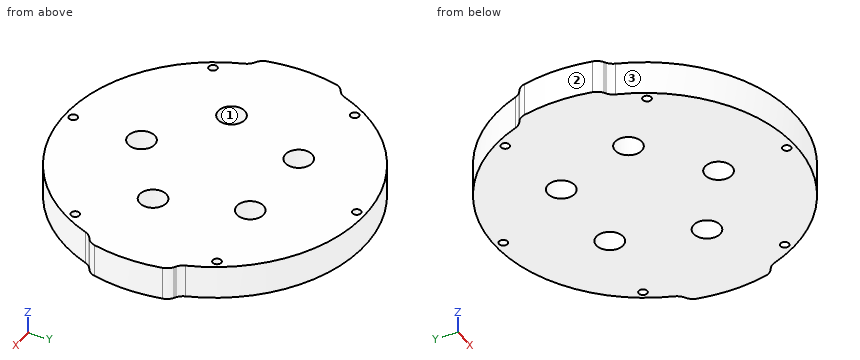
from build123d import *

# Parameters (mm, degrees)
SKETCH1_R           = 1.6
BOSS_EXTRUDE1_DEPTH = 12.7
SKETCH6_R           = 5.1
CUT_EXTRUDE2_DEPTH  = 13.7
FILLET1_R           = 5


with BuildPart() as part:
    # Sketch1 → Boss-Extrude1 (new body)
    with BuildSketch(Plane.XY):
        with BuildLine():
            Line((54.404710274, 17.5), (58.249656651, 15))
            ThreePointArc((58.249656651, 15), (60.15, 0), (58.249656651, -15))
            Line((58.249656651, -15), (54.404710274, -17.5))
            ThreePointArc((54.404710274, -17.5), (0, -57.15), (-54.404710274, -17.5))
            Line((-54.404710274, -17.5), (-58.249656651, -15))
            ThreePointArc((-58.249656651, -15), (-60.15, 0), (-58.249656651, 15))
            Line((-58.249656651, 15), (-54.404710274, 17.5))
            ThreePointArc((-54.404710274, 17.5), (0, 57.15), (54.404710274, 17.5))
        make_face()
        with Locations((0, 53.975)):
            Circle(SKETCH1_R, mode=Mode.SUBTRACT)
        with Locations((46.743721169, 26.9875)):
            Circle(SKETCH1_R, mode=Mode.SUBTRACT)
        with Locations((46.743721169, -26.9875)):
            Circle(SKETCH1_R, mode=Mode.SUBTRACT)
        with Locations((0, -53.975)):
            Circle(SKETCH1_R, mode=Mode.SUBTRACT)
        with Locations((-46.743721169, -26.9875)):
            Circle(SKETCH1_R, mode=Mode.SUBTRACT)
        with Locations((-46.743721169, 26.9875)):
            Circle(SKETCH1_R, mode=Mode.SUBTRACT)
    extrude(amount=BOSS_EXTRUDE1_DEPTH)

    # Sketch6 → Cut-Extrude2 (cut, through all)
    with BuildSketch(Plane(origin=(0, 0, 0), x_dir=(-1, 0, 0), z_dir=(0, 0, -1))):
        with Locations((16.457987064, 22.652475842)):
            Circle(SKETCH6_R)
        with Locations((-26.629582456, -8.652475842)):
            Circle(SKETCH6_R)
        with Locations((26.629582456, -8.652475842)):
            Circle(SKETCH6_R)
        with Locations((-16.457987064, 22.652475842)):
            Circle(SKETCH6_R)
        with Locations((0, -28)):
            Circle(SKETCH6_R)
    extrude(amount=-CUT_EXTRUDE2_DEPTH, mode=Mode.SUBTRACT)

    # Fillet1
    fillet1_edges = [part.edges().sort_by_distance(p)[0] for p in [
        (54.404710274, 17.5, 6.35),
        (58.249656651, 15, 6.35),
        (58.249656651, -15, 6.35),
        (54.404710274, -17.5, 6.35),
        (-54.404710274, -17.5, 6.35),
        (-58.249656651, -15, 6.35),
        (-58.249656651, 15, 6.35),
        (-54.404710274, 17.5, 6.35),
    ]]
    fillet(fillet1_edges, radius=FILLET1_R)


solid = part.part
Verification items for the finished model (mm, model axes). Face numbers are marked on the shaded views. Round coordinates to 2 decimals unless told otherwise and drop trailing zeros. Loops run counter-clockwise (first coordinate to the right, second up) from the corner with the lowest first, then second, coordinate; pieces in that order, holes last. Notation, with made-up numbers: (74, 69) - (97, 69) arc R13 cw to (97, 92) - close; hole circle Ø1 at (26, -25.75). An arc over 180 degrees is marked (long way). Use a Markdown table: item, result. Add a question column.
1. Thickness scan on probe 1 along Y at (x, z) = (0, 4.5) (3 decimals); probe 2 along Y at (x, z) = (-48, 2.5); probe 3 along X at (y, z) = (-7.5, 7.5). Record the ranges inside material, lowest first. Write a range as [from, to].
2. Gauge pin test, flat ends, axial feed: pin 1 (8 mm diameter, centred on x = 0, y = -28, fed in from -Z); pin 2 (16.5 mm diameter, centred on x = -16.46, y = 22.65, fed in from -Z); pin 3 (4 mm diameter, centred on y = -34, z = 3.5, fed in from -X); pin 4 (2 mm diameter, centred on y = -23, z = 10, fed in from -X). Record the tip position at first contact, or that the pin passes through.
3. Section check A-A, the plane x = 0. Record the boundary of the cut face in (y, z) (3 decimals).
4. Section check B-B, the plane x = 17.5. Record the boundary of the cut face in (y, z).
5. Section check C-C, the plane z = 6.75. Give the number of separate pieces and of enclosed holes in the cut face, plus the area to 3 significant figures.
6. Section check D-D, the plane y = 35.5. Record the boundary of the cut face in (x, z).
7. Release check for a two-part mould opening along Y. For the marked faces 1, 2 and 3 record: released by +Y, released by -Y, zero draft, split by the parting line, or undercut.
Checks:
| question | item | result |
|---|---|---|
| 1 | probe 1 | y = [-57.15, -55.575], [-52.375, -33.1], [-22.9, 52.375], [55.575, 57.15] |
| 1 | probe 2 | y = [-31.02, -27.98], [-26, 26], [27.98, 31.02] |
| 1 | probe 3 | x = [-59.68, -31.6], [-21.66, 21.66], [31.6, 59.68] |
| 2 | pin 1 | passes through |
| 2 | pin 2 | stops at z = 0 |
| 2 | pin 3 | stops at x = -47.35 |
| 2 | pin 4 | stops at x = -52.75 |
| 3 | outline | (-57.15, 0) - (-55.575, 0) - (-55.575, 12.7) - (-57.15, 12.7) - close; (-52.375, 0) - (-33.1, 0) - (-33.1, 12.7) - (-52.375, 12.7) - close; (-22.9, 0) - (52.375, 0) - (52.375, 12.7) - (-22.9, 12.7) - close; (55.575, 0) - (57.15, 0) - (57.15, 12.7) - (55.575, 12.7) - close |
| 4 | outline | (-54.4, 0) - (17.66, 0) - (17.66, 12.7) - (-54.4, 12.7) - close; (27.64, 0) - (54.4, 0) - (54.4, 12.7) - (27.64, 12.7) - close |
| 5 | separate pieces | 1 |
| 5 | enclosed holes | 11 |
| 5 | area | 10,000 mm^2 |
| 6 | outline | (-44.79, 0) - (44.79, 0) - (44.79, 12.7) - (-44.79, 12.7) - close |
| 7 | face 1 | undercut |
| 7 | face 2 | split by the parting line |
| 7 | face 3 | released by -Y |
